from build123d import *

# Parameters (mm, degrees)
F0_R     = 15
F1_DEPTH = 75
F3_DEPTH = 150
F4_W     = 23.585714
F4_H     = 7.8
F5_DEPTH = 21


with BuildPart() as f1:
    # F0 (on Front) → F1 (new body, symmetric)
    with BuildSketch(Plane.XZ):
        Circle(F0_R)
    extrude(amount=F1_DEPTH, both=True)

    # F2 (on face) → F3 (cut, symmetric)
    with BuildSketch(Plane.XZ.offset(75)):
        Polygon((-7.38566, -4.264113), (0, -8.528226), (7.38566, -4.264113), (7.38566, 4.264113), (0, 8.528226), (-7.38566, 4.264113), align=None)
    extrude(amount=F3_DEPTH, both=True, mode=Mode.SUBTRACT)

    # F4 (on Right) → F5 (cut, symmetric)
    with BuildSketch(Plane.YZ):
        Rectangle(F4_W, F4_H)
    extrude(amount=F5_DEPTH, both=True, mode=Mode.SUBTRACT)


solid = f1.part
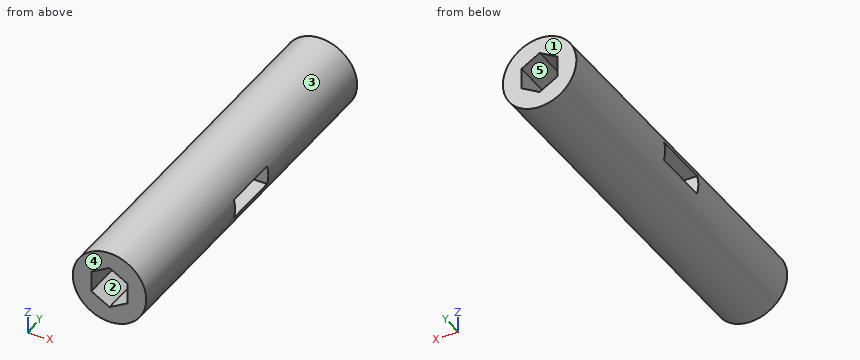
Check sheet for the modelled part. Datum: model origin and axes. Units: mm. Face numbers are marked on the shaded views. A direction names the side the tool comes from. Round coordinates to 2 decimals unless told otherwise and drop trailing zeros. Loops run counter-clockwise (first coordinate to the right, second up) from the corner with the lowest first, then second, coordinate; pieces in that order, holes last. Notation, with made-up numbers: M 14,56 L 56,56 A21 cw 56,70 Z; hole C -39.75,-33 d9. An arc over 180 degrees is marked long. One line per question, with ' | ' between items. Start each with the question number.
Item 1: Release check for a two-part mould opening along Z. For the marked faces 1, 2 and 3 record: released by +Z, released by -Z, zero draft, split by the parting line, or undercut.
Item 2: Scan lines: probe 1 along X at (y, z) = (-10.5, 4); probe 2 along X at (y, z) = (-32, 0.75); probe 3 along Z at (x, y) = (0, 1.5). Record each from-to range of solid material in increasing order.
Item 3: Section check D-D (z = -6.25). Record the boundary of the cut face in (x, y).
Item 4: Section check A-A (z = 0). Record the boundary of the cut face in (x, y), and give its area (3 significant figures).
Item 5: Section check B-B (y = 40). Record the boundary of the cut face in (x, z), and give its area (3 significant figures).
Item 6: Section check C-C (x = 3.5). Record the boundary of the cut face in (y, z), and give its area (3 significant figures).
Item 7: Set-up check for the marked faces 4 and 5: record each of +Z, -Z, +X, -X, +Y, -Y from which the full face is reachable in a straight line by a thin tool's end or side.
Item 8: Gauge pin test, flat ends, axial feed: pin 1 Ø2 at (x, y) = (-9.5, 5) entering from +Z; pin 2 Ø6 at (y, z) = (-32, -10) entering from +X; pin 3 Ø3.5 at (x, y) = (-10, -3) entering from -Z. Record the tip position at first contact, or that the pin passes through.
Worked out:
1) face 1: zero draft | face 2: undercut | face 3: split by the parting line
2) probe 1: -14.46 to -7.39, 7.39 to 14.46 | probe 2: -14.98 to -7.39, 7.39 to 14.98 | probe 3: -15 to -8.53, 8.53 to 15
3) outline: M -13.64,-75 L -3.95,-75 L -3.95,75 L -13.64,75 Z; M 3.95,-75 L 13.64,-75 L 13.64,75 L 3.95,75 Z
4) outline: M -15,-75 L -7.39,-75 L -7.39,-11.79 L -15,-11.79 Z; M -15,11.79 L -7.39,11.79 L -7.39,75 L -15,75 Z; M 7.39,-75 L 15,-75 L 15,-11.79 L 7.39,-11.79 Z; M 7.39,11.79 L 15,11.79 L 15,75 L 7.39,75 Z | area: 1,930 mm^2
5) outline: C 0,0 d30; hole M -7.39,-4.26 L 0,-8.53 L 7.39,-4.26 L 7.39,4.26 L 0,8.53 L -7.39,4.26 Z | area: 518 mm^2
6) outline: M -75,-14.59 L 75,-14.59 L 75,-6.51 L -75,-6.51 Z; M -75,6.51 L 75,6.51 L 75,14.59 L -75,14.59 Z | area: 2,420 mm^2
7) face 4: +Z, -Z, +X, -X, -Y | face 5: +Y, -Y
8) pin 1: z = 12.36 | pin 2: x = 13.27 | pin 3: z = -12.53
